Work out the finished part from the listing and answer in its coordinate system (mm). A direction names the side the tool comes from. Coordinates: 2 decimals unless noted, no trailing zeros. Loops run counter-clockwise (first coordinate to the right, second up) from the corner with the lowest first, then second, coordinate; pieces in that order, holes last. Notation, with made-up numbers: (31.25, 34) -> (89.25, 34) arc R37 ccw to (89.25, 71) -> close; hole circle Ø8 at (-14, 46). An arc over 180 degrees is marked (long way). One line per question, with ' | ' between items.
```python
from build123d import *

# Parameters (mm, degrees)
SKETCH1_W           = 200
SKETCH1_H           = 80
BOSS_EXTRUDE1_DEPTH = 10
SKETCH2_R           = 5
BOSS_EXTRUDE2_DEPTH = 160
SKETCH3_W           = 200
SKETCH3_H           = 80
BOSS_EXTRUDE3_DEPTH = 10
SKETCH7_R           = 20
CUT_EXTRUDE1_DEPTH  = 10


with BuildPart() as part:
    # Sketch1 → Boss-Extrude1 (new body)
    with BuildSketch(Plane.XY):
        Rectangle(SKETCH1_W, SKETCH1_H)
    extrude(amount=BOSS_EXTRUDE1_DEPTH)

    # Sketch2 → Boss-Extrude2 (add)
    with BuildSketch(Plane.XY):
        with Locations((-88.708175614, 29.131974832)):
            Circle(SKETCH2_R)
        with Locations((88.708175614, 29.131974832)):
            Circle(SKETCH2_R)
        with Locations((88.708175614, -29.131974832)):
            Circle(SKETCH2_R)
        with Locations((-88.708175614, -29.131974832)):
            Circle(SKETCH2_R)
    extrude(amount=BOSS_EXTRUDE2_DEPTH)

    # Sketch3 → Boss-Extrude3 (add)
    with BuildSketch(Plane.XY.offset(160)):
        Rectangle(SKETCH3_W, SKETCH3_H)
    extrude(amount=BOSS_EXTRUDE3_DEPTH)

    # Sketch7 → Cut-Extrude1 (cut)
    with BuildSketch(Plane.XY.offset(170)):
        Circle(SKETCH7_R)
        with Locations((-60, 0)):
            Circle(SKETCH7_R)
        with Locations((60, 0)):
            Circle(SKETCH7_R)
    extrude(amount=-CUT_EXTRUDE1_DEPTH, mode=Mode.SUBTRACT)


solid = part.part
```
1) Find section C-C (z = 120.5). Write down the section's boundary in (x, y), plus the area to 3 significant figures.
Check values:
outline: circle Ø10 at (-88.71, -29.13); circle Ø10 at (-88.71, 29.13); circle Ø10 at (88.71, -29.13); circle Ø10 at (88.71, 29.13) | area: 314 mm^2
2) Flat-ended cylindrical pins translate along their axes: pin 1 (4 mm diameter, centred on y = 25, z = 42, fed in from +X); pin 2 (12 mm diameter, centred on y = 25.5, z = 122, fed in from -X). Find the tip coordinate at first contact, or state that the pin passes through.
Check values:
pin 1: stops at x = 93.23 | pin 2: stops at x = -93.71
3) For faces 4 (the face through (-79.98, 0.88, 165.07)), 5 (the face through (83.713, 29.352, 83.95)), 6 (the face through (-100, -1, 5)), determine the directions among +Z, -Z, +X, -X, +Y, -Y from which every point of the face is accessible in a straight line to the end or side of a thin tool.
Check values:
face 4: +Z | face 5: none | face 6: +Z, -Z, -X, +Y, -Y
4) The mould has two halves that part along Y. Classify faces 1 (the face through (79.076, 6.007, 165.07)), 2 (the face through (-1, -40, 5)), 3 (the face through (-1, 40, 165)): released by +Y, released by -Y, zero draft, split by the parting line, or undercut.
Check values:
face 1: undercut | face 2: released by -Y | face 3: released by +Y
5) Find section A-A (x = 60). Write down the section's boundary in (y, z), plus the area to 3 significant figures.
Check values:
outline: (-40, 0) -> (40, 0) -> (40, 10) -> (-40, 10) -> close; (-40, 160) -> (-20, 160) -> (-20, 170) -> (-40, 170) -> close; (20, 160) -> (40, 160) -> (40, 170) -> (20, 170) -> close | area: 1,200 mm^2
6) Find section B-B (y = 3). Write down the section's boundary in (x, z).
Check values:
outline: (-100, 0) -> (100, 0) -> (100, 10) -> (-100, 10) -> close; (-100, 160) -> (-79.77, 160) -> (-79.77, 170) -> (-100, 170) -> close; (-40.23, 160) -> (-19.77, 160) -> (-19.77, 170) -> (-40.23, 170) -> close; (19.77, 160) -> (40.23, 160) -> (40.23, 170) -> (19.77, 170) -> close; (79.77, 160) -> (100, 160) -> (100, 170) -> (79.77, 170) -> close
7) Find the intervals of material crossed by line 1 along Z through (x, y) = (72, -27); line 2 along Y through (x, z) = (-60, 167.5); line 3 along Z through (x, y) = (19, 4.5), in increasing order.
Check values:
line 1: z = 0 to 10, 160 to 170 | line 2: y = -40 to -20, 20 to 40 | line 3: z = 0 to 10
